from build123d import *

# Parameters (mm, degrees)
CUT_EXTRUDE_1_DEPTH = 2


with BuildPart() as part:
    # Эскиз1 → Повернуть1 (revolve)
    with BuildSketch(Plane.XY, mode=Mode.PRIVATE) as revolve_1_sk:
        Polygon((0, 7.5), (7, 7.5), (7, 5.5), (4.85, 5.5), (4.85, 0), (0, 0), align=None)
    revolve(revolve_1_sk.sketch.rotate(Axis((0, 21.439331355, 0), (0, -1, 0)), 90), axis=Axis((0, 21.439331355, 0), (0, -1, 0)))

    # Эскиз2 → Вырез-Вытянуть1 (cut)
    with BuildSketch(Plane(origin=(0, 7.5, 0), x_dir=(1, 0, 0), z_dir=(0, 1, 0))):
        Polygon((2.309401077, 0), (1.154700538, 2), (-1.154700538, 2), (-2.309401077, 0), (-1.154700538, -2), (1.154700538, -2), align=None)
    extrude(amount=-CUT_EXTRUDE_1_DEPTH, mode=Mode.SUBTRACT)


solid = part.part
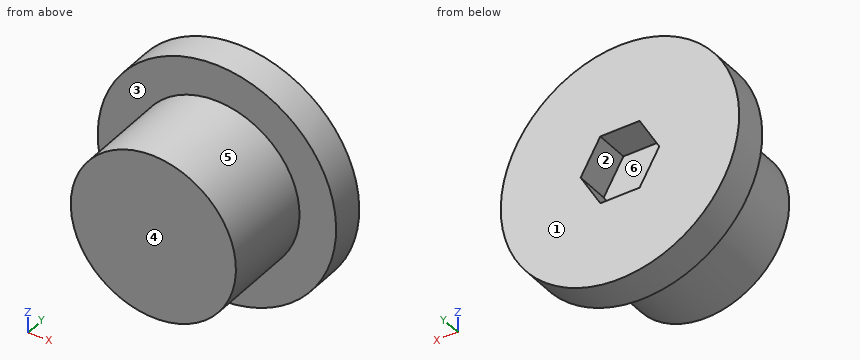
Part model, mm, in its own coordinate system. Face numbers are marked on the shaded views. A direction names the side the tool comes from. Coordinates: 2 decimals unless noted, no trailing zeros. Order: outer loops, then holes, each group sorted by start corner. A loop starts at its lowest first (then second) coordinate and runs counter-clockwise, first axis right, second up.
(1) Probe L1, parallel to Z at x = -0.75, y = 7; L2, parallel to Y at x = -2.5, z = -5.75; L3, parallel to X at y = 3.5, z = 0. List the from-to ranges inside material, lowest first.
Check sheet entries:
L1: z = -6.96 to -2, 2 to 6.96
L2: y = 5.5 to 7.5
L3: x = -4.85 to 4.85
(2) Slice it at D-D, the plane y = 2.25. Write the cut outline in (x, z).
Check sheet entries:
outline: circle Ø9.7 at (0, 0)
(3) Pin check, flat tips, straight feed: pin 1 Ø3 at (x, y) = (-3.5, 1) entering from +Z; pin 2 Ø4 at (x, y) = (2.5, 4) entering from -Z; pin 3 Ø3 at (y, z) = (4.5, 1.5) entering from -X. Stop position of each tip, or through.
Check sheet entries:
pin 1: stops at z = 4.42
pin 2: stops at z = -6.9
pin 3: stops at x = -6.99
(4) Pull direction Z, two halves, no side cores. Call the marked faces 4, 5 and 6: pulls with the +Z half, pulls with the -Z half, needs draft (parallel to the pull), parting line crosses it, or undercut.
Check sheet entries:
face 4: needs draft
face 5: parting line crosses it
face 6: undercut
(5) Slice it at B-B, the plane x = 0. Write the cut outline in (y, z).
Check sheet entries:
outline: (0, -4.85) - (5.5, -4.85) - (5.5, -7) - (7.5, -7) - (7.5, -2) - (5.5, -2) - (5.5, 2) - (7.5, 2) - (7.5, 7) - (5.5, 7) - (5.5, 4.85) - (0, 4.85) - close
(6) Slice it at A-A, the plane y = 6.75. Write the cut outline in (x, z), and give its area (3 significant figures).
Check sheet entries:
outline: circle Ø14 at (0, 0); hole (-2.31, 0) - (-1.15, -2) - (1.15, -2) - (2.31, 0) - (1.15, 2) - (-1.15, 2) - close
area: 140 mm2
(7) Slice it at C-C, the plane z = -2.75. Write the cut outline in (x, y) (3 decimals), and give its area (3 significant figures).
Check sheet entries:
outline: (-6.437, 5.5) - (-3.995, 5.5) - (-3.995, 0) - (3.995, 0) - (3.995, 5.5) - (6.437, 5.5) - (6.437, 7.5) - (-6.437, 7.5) - close
area: 69.7 mm2
(8) Tool access for the marked faces 1, 2 and 3: list every direction of +Z, -Z, +X, -X, +Y, -Y with a clear straight run to the whole face (end or side of a thin tool).
Check sheet entries:
face 1: +Z, -Z, +X, -X, +Y
face 2: +Y
face 3: -Y
